Could you check a few things on this model? Use its own coordinates, in mm. A direction names the side the tool comes from. Coordinates: 2 decimals unless noted, no trailing zeros. Order: outer loops, then holes, each group sorted by start corner. A loop starts at its lowest first (then second) coordinate and runs counter-clockwise, first axis right, second up. Notation, with made-up numbers: M -27.75,-28 L 14.25,-28 A34 cw 14.25,2 Z; hole C 39,87 d3. An arc over 180 degrees is marked long. Put each result on its own line as item: value. Start each with the question number.
```python
from build123d import *

# Parameters (mm, degrees)
SKETCH_2_W          = 4.013970818
SKETCH_2_H          = 10.71622578
SKETCH_2_W_2        = 3.089760279
SKETCH_2_H_2        = 12.863028926
CUT_EXTRUDE_1_DEPTH = 4
CUT_EXTRUDE_2_REACH = 14.427
SKETCH_3_R          = 1.25
SKETCH_3_W          = 1.5
SKETCH_3_H          = 2.5


with BuildPart() as part:
    # 草图1 → 旋转1 (revolve)
    with BuildSketch(Plane.XY, mode=Mode.PRIVATE) as revolve_1_sk:
        Polygon((7, -5.713091299), (7, -5.7), (7.75, -5.7), (8.5, -5.686908701), (8.5, -4.5), (6.5, -4.53491013), (6.5, -5), (0, -5.113457922), (0, -7.026182597), (3, -6.973817403), (3, -6.213444663), align=None)
    revolve(revolve_1_sk.sketch.rotate(Axis((-162.804450563, 0, 0), (1, 0, 0)), 270), axis=Axis((-162.804450563, 0, 0), (1, 0, 0)))  # turned: the seam where the file's is

    # 草图2 → 切除-拉伸1 (cut, through all)
    with BuildSketch(Plane(origin=(3, 0, 0), x_dir=(0, 0, -1), z_dir=(1, 0, 0))):
        with Locations((8.220430072, 0.592212477)):
            Rectangle(SKETCH_2_W, SKETCH_2_H)
        with Locations((-7.758324803, -0.481189096)):
            Rectangle(SKETCH_2_W_2, SKETCH_2_H_2)
    extrude(amount=-CUT_EXTRUDE_1_DEPTH, mode=Mode.SUBTRACT)

    # 切除-拉伸2: up to this cone (the profile starts outside it)
    cut_extrude_2_end = Plane(origin=(1.125, 0, 0), z_dir=(-1, 0, 0)) * Cone(4.737810595, 5.449831353, 40.791641948, mode=Mode.PRIVATE)
    # 草图3 → 切除-拉伸2 (cut, up to the surface)
    with BuildSketch(Plane.XY.offset(6.213444663), mode=Mode.PRIVATE) as cut_extrude_2_sk1:
        with Locations((1.5, 0)):
            Circle(SKETCH_3_R)
    cut_extrude_2_tool1 = extrude(cut_extrude_2_sk1.sketch, amount=-CUT_EXTRUDE_2_REACH, mode=Mode.PRIVATE) - cut_extrude_2_end
    add(cut_extrude_2_tool1.solids().sort_by_distance((1.5, 0, 6.213445))[0], mode=Mode.SUBTRACT)
    # 草图3 → 切除-拉伸2 (cut, up to the surface)
    with BuildSketch(Plane.XY.offset(6.213444663), mode=Mode.PRIVATE) as cut_extrude_2_sk2:
        with Locations((0.75, 0)):
            Rectangle(SKETCH_3_W, SKETCH_3_H)
    cut_extrude_2_tool2 = extrude(cut_extrude_2_sk2.sketch, amount=-CUT_EXTRUDE_2_REACH, mode=Mode.PRIVATE) - cut_extrude_2_end
    add(cut_extrude_2_tool2.solids().sort_by_distance((0.75, 0, 6.213445))[0], mode=Mode.SUBTRACT)


solid = part.part
```
Item 1: For pin 1 Ø2 at (x, y) = (6, 3) entering from -Z; pin 2 Ø1.5 at (x, y) = (4.5, 0) entering from +Z; pin 3 Ø1.5 at (x, z) = (1.5, 3) entering from -Y, each with a flat end and sliding along its axis, tell me the tip position at first contact or that it passes through.
Item 2: If we section it at A-A on x = 2: Write out the boundary of the cut face in (y, z), then the cut area to 3 significant figures.
Item 3: If we section it at B-B on x = 4.5: Write out the boundary of the cut face in (y, z).
Item 4: For faces 1 (the conical face through (7.49, -4.48, -0.59)), 2 (the flat face through (3, -6.3, -0.9)), 3 (the conical face through (8.21, 3.46, -4.52)), which set-ups out of +Z, -Z, +X, -X, +Y, -Y let a thin tool reach every point of the face, with its end or its side?
Item 5: I need wall thicknesses on probe 1 along X at (y, z) = (-6, -3); probe 2 along Z at (x, y) = (5.75, 3.25); probe 3 along X at (y, z) = (-3.5, 3.25). Which ranges of each line are inside material? Lowest first, please.
Item 6: If we mould it in two halves opening along Z, with no side actions, what happens to faces 4 (the flat face through (1, -1.25, 6)), 5 (the conical face through (3.204, -1.519, 4.824)), 6 (the conical face through (5.92, 5.71, -1.27))? For each: released by +Z, released by -Z, zero draft, split by the parting line, or undercut.
Geometry check:
1. pin 1: stops at z = -5.51
1. pin 2: stops at z = 6.12
1. pin 3: stops at y = -6.63
2. outline: M -3.2,-6.21 L 3.2,-6.21 A6.99 ccw 3.2,6.21 L 1.15,6.21 L 1.15,4.95 A5.08 cw long -1.15,4.95 L -1.15,6.21 L -3.2,6.21 A6.99 ccw Z
2. area: 63.1 mm²
3. outline: C 0,0 d12.05; hole C 0,0 d10.07
4. face 1: -X
4. face 2: +X, -Y
4. face 3: +X
5. probe 1: x = 0 to 3
5. probe 2: z = -4.89 to -3.82, 3.82 to 4.89
5. probe 3: x = 6.5 to 8.5
6. face 4: zero draft
6. face 5: undercut
6. face 6: split by the parting line
